Input: part model. Units: mm. Frame: model coordinates. Face numbers are marked on the shaded views. A direction names the side the tool comes from. Coordinates: 2 decimals unless noted, no trailing zeros. Order: outer loops, then holes, each group sorted by start corner. A loop starts at its lowest first (then second) coordinate and runs counter-clockwise, first axis right, second up. Notation, with made-up numbers: (-21.75, 3) -> (27.25, 3) arc R20 cw to (27.25, 15) -> close; hole circle Ø11 at (-25, 81). An arc over 180 degrees is marked (long way). Write each question's results on one line, items separated by ' | '.
```python
from build123d import *

# Parameters (mm, degrees)
PAD_DEPTH             = 10
POCKET_DEPTH          = 2
PAD001_DEPTH          = 28
PAD002_DEPTH          = 10
SKETCH004_R           = 16.5
POCKET001_DEPTH       = 0.5
SKETCH005_R           = 11
PAD003_DEPTH          = 2
SKETCH006_R           = 3.5
POCKET002_DEPTH       = 3
SKETCH007_R           = 1.5
POCKET003_DEPTH       = 5
POLARPATTERN_COUNT    = 4
SKETCH008_R           = 2.8
POCKET004_DEPTH       = 2
POLARPATTERN001_COUNT = 4
SKETCH009_R           = 3.25
POCKET005_DEPTH       = 3
SKETCH010_R           = 2.5
PAD004_DEPTH          = 1.3
CHAMFER_SIZE          = 0.5
SKETCH011_R           = 2.5
PAD005_DEPTH          = 25
CHAMFER001_SIZE       = 0.5
SKETCH012_W           = 30
SKETCH012_H           = 30
PAD006_DEPTH          = 0.1
POLARPATTERN002_COUNT = 2
SKETCH013_W           = 30
SKETCH013_H           = 30
PAD007_DEPTH          = 0.1
POLARPATTERN003_COUNT = 2


with BuildPart() as part:
    # Sketch → Pad (new body)
    with BuildSketch(Plane.XY):
        Polygon((-17, 20.213938), (17, 20.213938), (20.830222, 17), (20.830222, -17), (17, -20.213938), (-17, -20.213938), (-20.830222, -17), (-20.830222, 17), align=None)
    extrude(amount=PAD_DEPTH)

    # Sketch001 (on Face10 of Pad) → Pocket (cut)
    with BuildSketch(Plane.XY.offset(10)):
        Polygon((-20.830222, 15), (-15, 20.213938), (15, 20.213938), (20.830222, 15), (20.830222, -15), (15, -20.213938), (-15, -20.213938), (-20.830222, -15), align=None)
    extrude(amount=-POCKET_DEPTH, mode=Mode.SUBTRACT)

    # Sketch002 (on Face6 of Pocket) → Pad001 (join)
    with BuildSketch(Plane.XY.offset(8)):
        Polygon((-20.830222, 15), (-15, 20.213938), (15, 20.213938), (20.830222, 15), (20.830222, -15), (15, -20.213938), (-15, -20.213938), (-20.830222, -15), align=None)
    extrude(amount=PAD001_DEPTH)

    # Sketch003 (on Face12 of Pad001) → Pad002 (join)
    with BuildSketch(Plane.XY.offset(36)):
        Polygon((-20.830222, 17), (-17, 20.213938), (17, 20.213938), (20.830222, 17), (20.830222, -17), (17, -20.213938), (-17, -20.213938), (-20.830222, -17), align=None)
    extrude(amount=PAD002_DEPTH)

    # Sketch004 (on Face17 of Pad002) → Pocket001 (cut)
    with BuildSketch(Plane.XY.offset(46)):
        Circle(SKETCH004_R)
    extrude(amount=-POCKET001_DEPTH, mode=Mode.SUBTRACT)

    # Sketch005 (on Face28 of Pocket001) → Pad003 (join)
    with BuildSketch(Plane.XY.offset(45.5)):
        Circle(SKETCH005_R)
    extrude(amount=PAD003_DEPTH)

    # Sketch006 (on Face30 of Pad003) → Pocket002 (cut)
    with BuildSketch(Plane.XY.offset(47.5)):
        Circle(SKETCH006_R)
    extrude(amount=-POCKET002_DEPTH, mode=Mode.SUBTRACT)

    # Sketch007 (on Face14 of Pocket002) → Pocket003 (cut)
    with BuildSketch(Plane.XY.offset(46)):
        with Locations((-15.830222, 15.213938)):
            Circle(SKETCH007_R)
    pocket003 = extrude(amount=-POCKET003_DEPTH, mode=Mode.SUBTRACT)

    # PolarPattern: Pocket003 ×4 about axis
    polarpattern_axis = Axis((0, 0, 46), (0, 0, 1))
    for i in range(1, POLARPATTERN_COUNT):
        add(pocket003.rotate(polarpattern_axis, i * 360 / POLARPATTERN_COUNT), mode=Mode.SUBTRACT)

    # Sketch008 (on Face1 of PolarPattern) → Pocket004 (cut)
    with BuildSketch(Plane(origin=(0, 0, 0), x_dir=(1, 0, 0), z_dir=(0, 0, -1))):
        with Locations((-15.830222, 15.213938)):
            Circle(SKETCH008_R)
    pocket004 = extrude(amount=-POCKET004_DEPTH, mode=Mode.SUBTRACT)

    # PolarPattern001: Pocket004 ×4 about axis
    polarpattern001_axis = Axis((0, 0, 0), (0, 0, -1))
    for i in range(1, POLARPATTERN001_COUNT):
        add(pocket004.rotate(polarpattern001_axis, i * 360 / POLARPATTERN001_COUNT), mode=Mode.SUBTRACT)

    # Sketch009 (on Face1 of PolarPattern001) → Pocket005 (cut)
    with BuildSketch(Plane(origin=(0, 0, 0), x_dir=(1, 0, 0), z_dir=(0, 0, -1))):
        Circle(SKETCH009_R)
    extrude(amount=-POCKET005_DEPTH, mode=Mode.SUBTRACT)

    # Sketch010 (on Face33 of Pocket005) → Pad004 (join)
    with BuildSketch(Plane(origin=(0, 0, 3), x_dir=(1, 0, 0), z_dir=(0, 0, -1))):
        Circle(SKETCH010_R)
    extrude(amount=PAD004_DEPTH)

    # Chamfer
    chamfer_edges = [part.edges().sort_by_distance(p)[0] for p in [
        (-2.5, 0, 1.7),
    ]]
    chamfer(chamfer_edges, length=CHAMFER_SIZE)

    # Sketch011 (on Face53 of Chamfer) → Pad005 (join)
    with BuildSketch(Plane.XY.offset(44.5)):
        Circle(SKETCH011_R)
    extrude(amount=PAD005_DEPTH)

    # Chamfer001
    chamfer001_edges = [part.edges().sort_by_distance(p)[0] for p in [
        (-2.5, 0, 69.5),
    ]]
    chamfer(chamfer001_edges, length=CHAMFER001_SIZE)

    # Sketch012 (on Face16 of Chamfer001) → Pad006 (join)
    with BuildSketch(Plane.XZ.offset(20.213938)):
        with Locations((0, 23)):
            Rectangle(SKETCH012_W, SKETCH012_H)
    pad006 = extrude(amount=PAD006_DEPTH)

    # PolarPattern002: Pad006 ×2 about axis
    polarpattern002_axis = Axis((0, 0, 0), (0, 0, -1))
    for i in range(1, POLARPATTERN002_COUNT):
        add(pad006.rotate(polarpattern002_axis, i * 360 / POLARPATTERN002_COUNT))

    # Sketch013 (on Face17 of PolarPattern002) → Pad007 (join)
    with BuildSketch(Plane.YZ.offset(20.830222)):
        with Locations((0, 23)):
            Rectangle(SKETCH013_W, SKETCH013_H)
    pad007 = extrude(amount=PAD007_DEPTH)

    # PolarPattern003: Pad007 ×2 about axis
    polarpattern003_axis = Axis((0, 0, 0), (0, 0, 1))
    for i in range(1, POLARPATTERN003_COUNT):
        add(pad007.rotate(polarpattern003_axis, i * 360 / POLARPATTERN003_COUNT))


solid = part.part
```
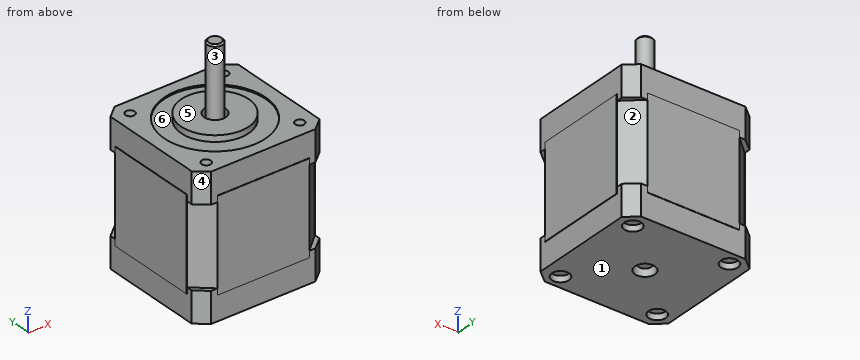
(1) Cut plane B-B, the plane x = 8. Return loops of the section in (y, z), plus the area to 3 significant figures.
Return value:
outline: (-20.31, 8) -> (-20.21, 8) -> (-20.21, 0) -> (20.21, 0) -> (20.21, 8) -> (20.31, 8) -> (20.31, 38) -> (20.21, 38) -> (20.21, 46) -> (14.43, 46) -> (14.43, 45.5) -> (7.55, 45.5) -> (7.55, 47.5) -> (-7.55, 47.5) -> (-7.55, 45.5) -> (-14.43, 45.5) -> (-14.43, 46) -> (-20.21, 46) -> (-20.21, 38) -> (-20.31, 38) -> close | area: 1,880 mm2
(2) Line query: line 1 along Z through (x, y) = (10, -12); line 2 along Z through (x, y) = (17, 13); line 3 along X through (y, z) = (-5, 39). Output: solid intervals per line, ascending. Write a range as from..to.
Return value:
line 1: 0..45.5 | line 2: 2..46 | line 3: -20.83..20.83
(3) Cut plane C-C, the plane z = 53. Return loops of the section in (x, y), plus the area to 3 significant figures.
Return value:
outline: circle Ø5 at (0, 0) | area: 19.6 mm2
(4) Cut plane A-A, the plane z = 30.5. Return loops of the section in (x, y), plus the area to 3 significant figures.
Return value:
outline: (-20.93, -15) -> (-20.83, -15) -> (-15, -20.21) -> (-15, -20.31) -> (15, -20.31) -> (15, -20.21) -> (20.83, -15) -> (20.93, -15) -> (20.93, 15) -> (20.83, 15) -> (15, 20.21) -> (15, 20.31) -> (-15, 20.31) -> (-15, 20.21) -> (-20.83, 15) -> (-20.93, 15) -> close | area: 1,640 mm2
(5) Reachability of the marked faces 1, 2 and 3 from +Z, -Z, +X, -X, +Y, -Y: full face, straight path, thin tool, end or side. Return the list, or none.
Return value:
face 1: -Z, +X, -X, +Y, -Y | face 2: +X, +Y | face 3: +Z
(6) Mould query, pull axis X, two halves, no side actions, for the marked faces 4, 5 and 6. Classes: +X half, -X half, draft (parallel to the pull), parting line (faces both ways), or undercut.
Return value:
face 4: -X half | face 5: draft | face 6: undercut
(7) Pin query (flat end, axial travel): P1, Ø5, axis at y = 5, z = 42.5, coming from the -X side; P2, Ø4, axis at x = 17.5, y = 17.5, coming from the +Z side; P3, Ø2.5, axis at x = -17, y = 18, coming from the -Z side; P4, Ø5, axis at x = 7, z = 45, coming from the +Y side. Return the tip coordinate at first contact, or that it passes through.
Return value:
P1: x = -20.83 | P2: z = 46 | P3: z = 0 | P4: y = 20.21
